Design review of the part built by this model. Coordinates are the model's own, in mm. A direction names the side the tool comes from. Coordinates: 2 decimals unless noted, no trailing zeros. Loops run counter-clockwise (first coordinate to the right, second up) from the corner with the lowest first, then second, coordinate; pieces in that order, holes last. Notation, with made-up numbers: (33.25, 29.25) - (87.25, 29.25) arc R14 ccw to (87.25, 50.25) - close; hole circle Ø1 at (-13.5, 79). An arc over 180 degrees is marked (long way). Use one line per item in the form item = value. Start each with the question number.
(1) The part is to be moulded in two halves that separate along Z. For faces 3 (the face through (14.901, 5, 42)), 4 (the face through (11, 11, 63.5)), 5 (the face through (22.352, 11, 32)), say which applies: pulls with the +Z half, pulls with the -Z half, needs draft (parallel to the pull), parting line crosses it, or undercut.
(2) Add section B-B (y = 1.5). State the section outline as (x, z) points.
(3) Tool access review of faces 1 (the face through (0, 11, 31)), 2 (the face through (11, 9, 50.8)): name each direction out of +Z, -Z, +X, -X, +Y, -Y from which nothing blocks a thin tool from reaching the whole face with its end or side.
(4) Add section C-C (z = 42.5). State the section outline as (x, y) points.
(5) Add section D-D (y = 10.25). State the section outline as (x, z) points.
(6) Clearance check with a flat-ended pin moving along its axis: pin 1 Ø5 at (x, z) = (11.5, 36.5) entering from -Y. State where the tip first meets the part, or that it passes through.
(7) For L1, parallel to Z at x = 13, y = 12; L2, parallel to Z at x = 10, y = 5.75; L3, parallel to Y at x = 13.75, z = 49.5, list the stretches that pass through material, from the lowest coordinate up.
(8) Add section A-A (x = 12.75). State the section outline as (y, z) points.
Autodesk Fusion 360 part; units mm, degrees
sketch "Sketch1" plane through (0, 0, 0) normal (0, 0, 1) x (1, 0, 0)
  line L0 (0, 0) -> (22.352, 0)
  line L1 (22.352, 0) -> (22.352, 22.352)
  line L2 (22.352, 22.352) -> (0, 22.352)
  line L3 (0, 22.352) -> (0, 0)
  line L4 (7.4507, 22.352) -> (7.4507, 0)
  dimension "d1" = 22.352
  dimension "d2" = 22.352
  dimension "d3" = 7.4507
extrude "Extrude1" add sketch "Sketch1" along normal blind 63.5 contours L0 L2 L3 L4
sketch "Sketch2" plane through (7.4507, 0, 0) normal (1, 0, 0) x (0, 0, -1)
  line L0 (0, 0) -> (0, 22.352)
  line L1 (0, 22.352) -> (-63.5, 22.352)
  line L2 (-63.5, 22.352) -> (-63.5, 0)
  line L3 (-63.5, 0) -> (0, 0)
  line L4 (-50.8, 0) -> (-50.8, 19.1554)
  line L5 (-50.8, 19.1554) -> (-17.6219, 0)
  dimension "d6" = 12.7
  dimension "d7" = 30
extrude "Extrude2" add sketch "Sketch2" along normal blind 7.4507 contours L0 L1 L2 L3 L4 L5
sketch "Sketch3" plane through (14.9013, 0, 0) normal (1, 0, 0) x (0, 0, -1)
  line L0 (-50.8, 19.1554) -> (-17.6219, 0)
  line L1 (-17.6219, 0) -> (0, 0)
  line L2 (0, 0) -> (0, 22.352)
  line L3 (0, 22.352) -> (-63.5, 22.352)
  line L4 (-63.5, 22.352) -> (-63.5, 0)
  line L5 (-63.5, 0) -> (-50.8, 0)
  line L6 (-50.8, 0) -> (-50.8, 19.1554)
  line L7 (-63.5, 0) -> (0, 0)
  line L8 (0, 0) -> (0, 22.352)
  line L9 (0, 22.352) -> (-63.5, 22.352)
  line L10 (-63.5, 22.352) -> (-63.5, 0)
extrude "Extrude3" add sketch "Sketch3" along normal blind 7.4507
equation "d3 = ( 0.88 / 3 ) * 1 in"
equation "d8 = ( 0.88 / 3 ) * 1 in"
equation "d10 = ( 0.88 / 3 ) * 1 in"
Computed values:
q1.face_3 = undercut
q1.face_4 = pulls with the +Z half
q1.face_5 = needs draft
q2.outline = (0, 0) - (22.35, 0) - (22.35, 63.5) - (0, 63.5) - close; hole (7.45, 20.22) - (14.9, 20.22) - (14.9, 50.8) - (7.45, 50.8) - close
q3.face_1 = +Z, -Z, -X, +Y, -Y
q3.face_2 = -Y
q4.outline = (0, 0) - (7.45, 0) - (7.45, 14.36) - (14.9, 14.36) - (14.9, 0) - (22.35, 0) - (22.35, 22.35) - (0, 22.35) - close
q5.outline = (0, 0) - (22.35, 0) - (22.35, 63.5) - (0, 63.5) - close; hole (7.45, 35.38) - (14.9, 35.38) - (14.9, 50.8) - (7.45, 50.8) - close
q6.pin_1 = 9.46
q7.L1 = 0 to 38.41, 50.8 to 63.5
q7.L2 = 0 to 27.58, 50.8 to 63.5
q7.L3 = 18.4 to 22.35
q8.outline = (0, 0) - (22.35, 0) - (22.35, 63.5) - (0, 63.5) - (0, 50.8) - (19.16, 50.8) - (0, 17.62) - close
